Autodesk Inventor part; units mm, degrees
ref_plane "YZ Plane" through (0, 0, 0) normal (1, 0, 0) x (0, 1, 0)
ref_plane "XZ Plane" through (0, 0, 0) normal (0, 1, 0) x (-1, 0, 0)
sketch "Эскиз1" plane through (0, 0, 0) normal (1, 0, 0) x (0, 1, 0)
  line L0 (0, 0) -> (0, 11.5)
  line L1 (0, 11.5) -> (0, 13.5)
  line L2 (0, 13.5) -> (2, 13.5)
  line L3 (2, 13.5) -> (0, 11.5)
  line L4 (2, 13.5) -> (6.5, 13.5)
  line L5 (6.5, 13.5) -> (6.5, 16.5)
  line L6 (6.5, 16.5) -> (2, 16.5)
  line L7 (0, 13.5) -> (0, 16.5)
  line L8 (0, 16.5) -> (2, 16.5)
  line L9 (6.5, 16.5) -> (-10, 33)
  line L10 (6.5, 16.5) -> (32.9156, 16.5) construction
  line L11 (0, 33) -> (-10, 33)
  line L12 (-10, 33) -> (-10, 16.5)
  line L13 (-10, 16.5) -> (-9.9702, 14.7974) construction
  line L14 (-9.9702, 14.7974) -> (-9.629, 12.8623) construction
  line L15 (-9.629, 12.8623) -> (-8.0037, 11.5) construction
  line L16 (-8.0037, 11.5) -> (0, 11.5) construction
  spline S0 degree 4 poles (-10, 16.5) (-9.9702, 14.7974) (-9.629, 12.8623) (-8.0037, 11.5) (0, 11.5) knots 1 1 1 1 1 2 2 2 2 2
  line L17 (0, 0) -> (14.3588, 0)
  dimension "d1" = 2
  dimension "d2" = 2
  dimension "d3" = 13.5
  dimension "d4" = 3
  dimension "d5" = 4.5
  dimension "d6" = 16.5
  dimension "d7" = 135
revolve "Вращение1" add sketch "Эскиз1" angle 360 about axis through (0, 0, 0) along (0, 1, 0)
sketch "Эскиз2" plane through (0, 0, 0) normal (0, 0, 1) x (1, 0, 0)
  line L0 (13.5, 6.5) -> (-13.5, 6.5)
  line L1 (13.5, 2) -> (-13.5, 2)
  line L2 (0, 2) -> (0, 6.5)
  circle A0 centre (0, 4.25) radius 1
  point P0 (0, 0)
  dimension "d9" = 2
extrude "Выдавливание1" cut sketch "Эскиз2" along normal blind 30
ref_plane "РабПлоскость1" through (0, 0, 36.5125) normal (0, 0, 1) x (1, 0, 0)
sketch "Эскиз3" plane through (0, 0, 36.5125) normal (0, 0, 1) x (1, 0, 0)
  line L0 (16.5, 6.5) -> (-16.5, 6.5)
  arc A0 (-2, 4.25) -> (2, 4.25) centre (0, 4.25) ccw
  line L1 (-2, 4.25) -> (-2, 6.5)
  line L2 (2, 4.25) -> (2, 6.5)
  point P0 (0, 0)
  point P1 (0.9986, 4.3033)
  dimension "d14" = 4
extrude "Выдавливание2" cut sketch "Эскиз3" against normal blind 20.013
pattern_circular "Круговой массив1" count 4 over 360 about axis through (0, 4.25, 0) along (0, 1, 0) of "Выдавливание2", "Выдавливание1"
properties part number "Статор без зубьев"
Verification items for the finished model (mm, model axes). A direction names the side the tool comes from. Give positions to 0.01 mm unless a question says otherwise; leave off trailing zeros. Write item = value, one per line.
(1) Go/stop test with flat-tipped pins: pin 1 Ø1.8 at (y, z) = (4.25, 0) entering from -X; pin 2 Ø2.5 at (x, y) = (0, 4.25) entering from -Z; pin 3 Ø1.2 at (x, y) = (-0.5, 4.5) entering from +Z; pin 4 Ø8 at (x, z) = (-9.5, -21) entering from +Y. Record where each tip stops, or that it passes through.
Found:
pin_1 = through
pin_2 = -16.5
pin_3 = 16.5
pin_4 = 3.95
(2) Material ranges on line 1 (X direction, y = 5.6, z = 0); line 2 (Y direction, x = 0, z = -14.1); line 3 (Z direction, x = -2, y = -5.5), recorded low to high.
Found:
line_1 = -16.5 to -13.5, 13.5 to 16.5
line_2 = -9.51 to 3.25, 5.25 to 6.5
line_3 = -28.43 to -11.71, 11.71 to 28.43
(3) Access from +Z, -Z, +X, -X, +Y, -Y to the whole of each face (thin tool, end or side, straight path). Record for faces 1 (the face through (-14.96, 3.26, -0.13)), 2 (the face through (2, 5, -17)), 3 (the face through (-0.5, 5.3, 16.5)), 4 (the face through (-18.18, 2.25, -0.04)), 5 (the face through (16.5, 5.3, 0.5)).
Found:
face_1 = +X, -X
face_2 = -Z, +Y
face_3 = +Z, +Y
face_4 = -X, +Y
face_5 = +X, +Y
(4) Draft check along Z on faces 6 (the face through (17, 5, 2)), 7 (the face through (-5.27, 5.47, 16.72)), 8 (the face through (17, 5, -2)), 9 (the face through (-2, 5, 17)). Enter one of: released by +Z, released by -Z, zero draft, split by the parting line, or undercut.
Found:
face_6 = undercut
face_7 = split by the parting line
face_8 = undercut
face_9 = zero draft
